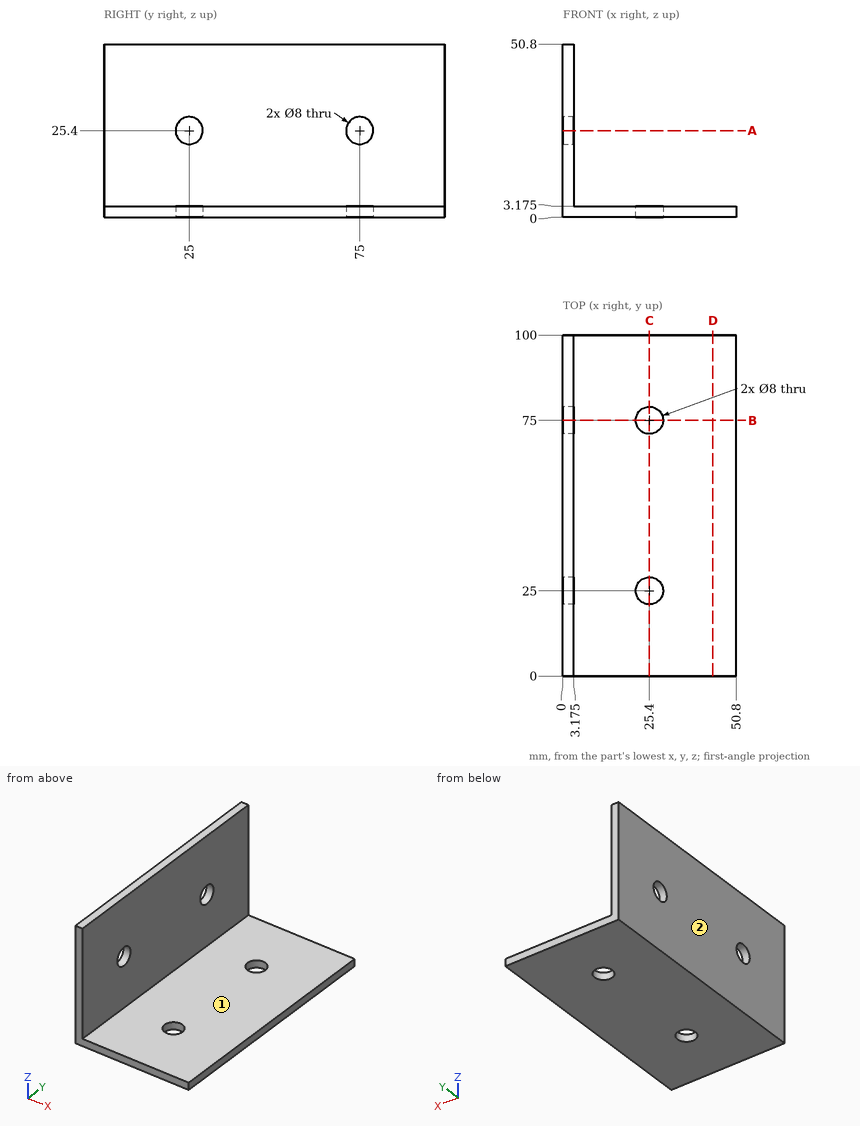
For this review, use the dimensioned drawing (mm, ordinates from the lowest corner) and the shaded views. A direction names the side the tool comes from. Coordinates: 2 decimals unless noted, no trailing zeros. Write each loop counter-clockwise with the first axis right and the second up, starting at its lowest first coordinate (ties: lowest second). Pieces come first, ordered by that corner, then holes. Notation, with made-up numbers: (63.25, -0.75) - (73.25, -0.75) arc R30 cw to (73.25, 25.25) - close; hole circle Ø9 at (66, 13.25). An arc over 180 degrees is marked (long way). Answer as a JSON object with one key per item and string values. Group by question number.
1. Machinability: for the marked faces 1 and 2, which of the approach directions +Z, -Z, +X, -X, +Y, -Y give a long, thin tool a straight path to every point of the face, cutting with its end or side? Answer none if there is none.
2. Add section C-C (x = 25.4). Give the boundary of the cut face in (y, z) (3 decimals), plus the area to 3 significant figures.
3. Clearance check with flat-ended pins moving along their axes: pin 1 Ø5 at (x, y) = (23.5, 76) entering from -Z; pin 2 Ø1.5 at (x, y) = (7.5, 85) entering from +Z (3 decimals); pin 3 Ø13 at (y, z) = (75, 25.4) entering from +X (3 decimals). State where each tip first meets the part, or that it passes through.
4. Add section B-B (y = 75). Give the boundary of the cut face in (x, z) (3 decimals), plus the area to 3 significant figures.
5. Add section D-D (x = 44). Give the boundary of the cut face in (y, z) (3 decimals), plus the area to 4 significant figures.
6. Add section A-A (z = 25.4). Give the boundary of the cut face in (x, y) (3 decimals).
7. To check wall thickness, follow probe 1 along Y at (x, z) = (25.4, 0.7); probe 2 along X at (y, z) = (86, 23.5) (3 decimals). State the ranges of each line that lie inside material, in increasing order.
Findings:
{
 "1": {"face 1": "+Z, +X, +Y, -Y", "face 2": "+Z, -Z, -X, +Y, -Y"},
 "2": {"outline": "(0, 0) - (21, 0) - (21, 3.175) - (0, 3.175) - close; (29, 0) - (71, 0) - (71, 3.175) - (29, 3.175) - close; (79, 0) - (100, 0) - (100, 3.175) - (79, 3.175) - close", "area": "267 mm²"},
 "3": {"pin 1": "z = 0", "pin 2": "z = 3.175", "pin 3": "x = 3.175"},
 "4": {"outline": "(0, 0) - (21.4, 0) - (21.4, 3.175) - (3.175, 3.175) - (3.175, 21.4) - (0, 21.4) - close; (0, 29.4) - (3.175, 29.4) - (3.175, 50.8) - (0, 50.8) - close; (29.4, 0) - (50.8, 0) - (50.8, 3.175) - (29.4, 3.175) - close", "area": "262 mm²"},
 "5": {"outline": "(0, 0) - (100, 0) - (100, 3.175) - (0, 3.175) - close", "area": "317.5 mm²"},
 "6": {"outline": "(0, 0) - (3.175, 0) - (3.175, 21) - (0, 21) - close; (0, 29) - (3.175, 29) - (3.175, 71) - (0, 71) - close; (0, 79) - (3.175, 79) - (3.175, 100) - (0, 100) - close"},
 "7": {"probe 1": "0 to 21, 29 to 71, 79 to 100", "probe 2": "0 to 3.175"}
}
